from build123d import *

# Parameters (mm, degrees)
SKETCH1_W           = 1240
SKETCH1_H           = 505
BOSS_EXTRUDE1_DEPTH = 10
SKETCH2_W           = 1100
SKETCH2_H           = 400
CUT_EXTRUDE1_DEPTH  = 670.519417194
SKETCH3_W           = 1120
SKETCH3_H           = 420
CUT_EXTRUDE2_DEPTH  = 5


with BuildPart() as part:
    # Sketch1 → Boss-Extrude1 (new body)
    with BuildSketch(Plane(origin=(0, 0, 0), x_dir=(1, 0, 0), z_dir=(0, 1, 0))):
        Rectangle(SKETCH1_W, SKETCH1_H)
    extrude(amount=BOSS_EXTRUDE1_DEPTH)

    # Sketch2 → Cut-Extrude1 (cut, through all)
    with BuildSketch(Plane(origin=(0, 10, 0), x_dir=(1, 0, 0), z_dir=(0, 1, 0))):
        Rectangle(SKETCH2_W, SKETCH2_H)
    extrude(amount=-CUT_EXTRUDE1_DEPTH, mode=Mode.SUBTRACT)

    # Sketch3 → Cut-Extrude2 (cut)
    with BuildSketch(Plane(origin=(0, 10, 0), x_dir=(1, 0, 0), z_dir=(0, 1, 0))):
        Rectangle(SKETCH3_W, SKETCH3_H)
    extrude(amount=-CUT_EXTRUDE2_DEPTH, mode=Mode.SUBTRACT)


solid = part.part
The model under review builds one solid part; all positions refer to its coordinate system, in mm. Round coordinates to 2 decimals unless told otherwise and drop trailing zeros. Loops run counter-clockwise (first coordinate to the right, second up) from the corner with the lowest first, then second, coordinate; pieces in that order, holes last. Notation, with made-up numbers: (62.25, 84) -> (115.25, 84) arc R22 ccw to (115.25, 91) -> close; hole circle Ø9 at (31.25, -28). An arc over 180 degrees is marked (long way). Return JSON: item names as keys, results as strings.
(1) For pin 1 (2 mm diameter, centred on x = 349, z = 202, fed in from +Y), flat-tipped, find the tip position at first contact; note if it passes through.
Solved:
{"pin 1": "y = 5"}
(2) Add section B-B on y = 7.25. Write out the cut boundary in (x, z), plus the area to 3 significant figures.
Solved:
{"outline": "(-620, -252.5) -> (620, -252.5) -> (620, 252.5) -> (-620, 252.5) -> close; hole (-560, -210) -> (560, -210) -> (560, 210) -> (-560, 210) -> close", "area": "156,000 mm2"}
(3) For line 1 (Z direction, x = 509.5, y = 5.5); line 2 (X direction, y = 7.25, z = -103); line 3 (Z direction, x = -522, y = 0.75), list the stretches that pass through material, from the lowest coordinate up.
Solved:
{"line 1": "-252.5 to -210, 210 to 252.5", "line 2": "-620 to -560, 560 to 620", "line 3": "-252.5 to -200, 200 to 252.5"}
(4) Add section A-A on z = 123.5. Write out the cut boundary in (x, y), plus the area to 3 significant figures.
Solved:
{"outline": "(-620, 0) -> (-550, 0) -> (-550, 5) -> (-560, 5) -> (-560, 10) -> (-620, 10) -> close; (550, 0) -> (620, 0) -> (620, 10) -> (560, 10) -> (560, 5) -> (550, 5) -> close", "area": "1,300 mm2"}
(5) The part is to be moulded in two halves that separate along X. For faces 1 (the flat face through (-3, 5, -203)), 2 (the flat face through (-49, 10, 223)), say which applies: released by +X, released by -X, zero draft, split by the parting line, or undercut.
Solved:
{"face 1": "undercut", "face 2": "zero draft"}
(6) Add section C-C on x = 70. Write out the cut boundary in (y, z).
Solved:
{"outline": "(0, -252.5) -> (10, -252.5) -> (10, -210) -> (5, -210) -> (5, -200) -> (0, -200) -> close; (0, 200) -> (5, 200) -> (5, 210) -> (10, 210) -> (10, 252.5) -> (0, 252.5) -> close"}
